Design review of the part shown in the three views and the two pictorial views. Dimensions are in mm from the part's minimum x, y and z. Give positions to 0.01 mm unless a question says otherwise; leave off trailing zeros. Order: outer loops, then holes, each group sorted by start corner. A loop starts at its lowest first (then second) coordinate and runs counter-clockwise, first axis right, second up. Notation, with made-up numbers: M 52,-10 L 76,-10 A24 cw 76,22 Z; hole C -20,17 d7. An arc over 180 degrees is marked long. Answer as a JSON object with one key per item and string values.
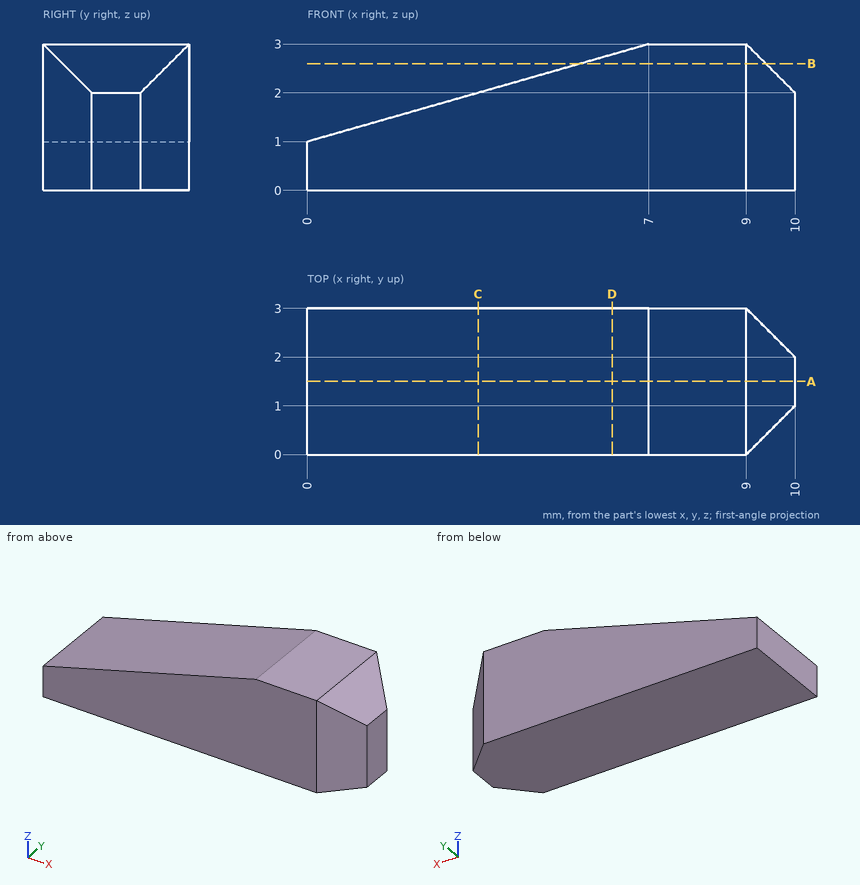
(1) We need section D-D (x = 6.25). Write out the cut boundary in (y, z), plus the area to 3 significant figures.
Checked values:
{"outline": "M 0,0 L 3,0 L 3,2.79 L 0,2.79 Z", "area": "8.36 mm^2"}
(2) We need section C-C (x = 3.5). Write out the cut boundary in (y, z).
Checked values:
{"outline": "M 0,0 L 3,0 L 3,2 L 0,2 Z"}
(3) We need section A-A (y = 1.5). Write out the cut boundary in (x, z), plus the area to 3 significant figures.
Checked values:
{"outline": "M 0,0 L 10,0 L 10,2 L 9,3 L 7,3 L 0,1 Z", "area": "22.5 mm^2"}
(4) Insertion check: pin 1 (1 mm diameter, centred on y = 1.5, z = 1, fed in from -X); pin 2 (1 mm diameter, centred on x = 2.5, y = 2.5, fed in from +Z). Each pin has a flat end and moves straight along its axis. Give the tip position at first contact, or say it passes through.
Checked values:
{"pin 1": "stops at x = 0", "pin 2": "stops at z = 1.86"}
(5) We need section B-B (z = 2.6). Write out the cut boundary in (x, y), plus the area to 3 significant figures.
Checked values:
{"outline": "M 5.6,0 L 9,0 L 9.4,0.4 L 9.4,2.6 L 9,3 L 5.6,3 Z", "area": "11.2 mm^2"}
(6) To check wall thickness, follow L1, parallel to Z at x = 0.75, y = 2.3; L2, parallel to Z at x = 2, y = 1.3; L3, parallel to Y at x = 9.25, z = 1.25. State the ranges of each line that lie inside material, in increasing order. Write a range as from..to.
Checked values:
{"L1": "z = 0..1.21", "L2": "z = 0..1.57", "L3": "y = 0.25..2.75"}
